Part print with two shaded views. Sizes in mm from the minimum x, y, z corner. A direction names the side the tool comes from. Coordinates: 2 decimals unless noted, no trailing zeros. Loops run counter-clockwise (first coordinate to the right, second up) from the corner with the lowest first, then second, coordinate; pieces in that order, holes last.
(1) Slice it at C-C (z = 13.75). Give the cut face in (x, y).
(2) Two-plate mould, pull along X, no slides. Class the marked faces 3, 4 and 5: pulls with the +X half, pulls with the -X half, needs draft (parallel to the pull), parting line crosses it, or undercut.
(3) Slice it at B-B (y = 1.25). Give the cut face in (x, z) (3 decimals).
(4) Slice it at A-A (x = 66.5). Give the cut face in (y, z).
(5) Tool access for the marked faces 1 and 2: list every direction of +Z, -Z, +X, -X, +Y, -Y with a clear straight run to the whole face (end or side of a thin tool).
(6) Wall check: L1, parallel to Z at x = 66.5, y = 2; L2, parallel to X at y = 6.25, z = 8.75; L3, parallel to X at y = 1, z = 7.75. Give the ranges that are in metal, low to high.
(7) Flat gauge pin, fed straight in: P1, Ø4, axis at x = 9.35, z = 9.525, coming from the +Y side. Where does the tip first touch, or does it go through?
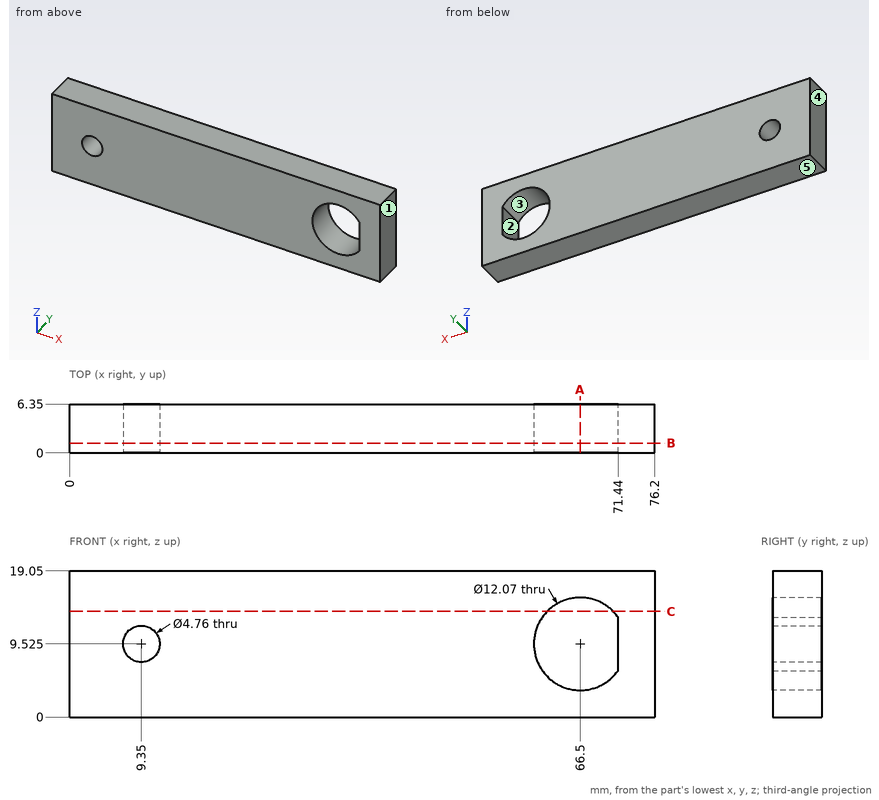
Response values:
1. outline: (0, 0) - (62.19, 0) - (62.19, 6.35) - (0, 6.35) - close; (70.81, 0) - (76.2, 0) - (76.2, 6.35) - (70.81, 6.35) - close
2. face 3: undercut
2. face 4: pulls with the -X half
2. face 5: needs draft
3. outline: (0, 0) - (76.2, 0) - (76.2, 19.05) - (0, 19.05) - close; hole circle Ø4.76 at (9.35, 9.525); hole (71.44, 6.058) - (71.44, 12.992) arc R6.035 ccw (long way) to start
4. outline: (0, 0) - (6.35, 0) - (6.35, 3.49) - (0, 3.49) - close; (0, 15.56) - (6.35, 15.56) - (6.35, 19.05) - (0, 19.05) - close
5. face 1: +Z, -Z, +X, +Y, -Y
5. face 2: +Y, -Y
6. L1: z = 0 to 3.49, 15.56 to 19.05
6. L2: x = 0 to 7.1, 11.6 to 60.51, 71.44 to 76.2
6. L3: x = 0 to 7.76, 10.94 to 60.73, 71.44 to 76.2
7. P1: passes through
